Could you check a few things on this drawing? It's one solid part, dimensions in mm from its lowest x, y, z. A direction names the side the tool comes from. Round coordinates to 2 decimals unless told otherwise and drop trailing zeros. Write each loop counter-clockwise with the first axis right and the second up, starting at its lowest first coordinate (ties: lowest second). Pieces come first, ordered by that corner, then holes. Notation, with made-up numbers: M -3,-31 L 46,-31 A16 ccw 46,-16 Z; hole C 46,61 d10. An arc over 180 degrees is marked long. One line per item, written item: value. Start each with the question number.
(1) I want a section at C-C on y = 6. Please give me the cut outline in (x, z), and give its area (3 significant figures).
(2) Thinking about a two-plate mould opening in Z: for the marked faces 1, 2 and 3, which applies, released by +Z, released by -Z, zero draft, split by the parting line, or undercut?
(3) I want a section at B-B on z = 0.5. Please give me the cut outline in (x, y).
(4) I want a section at A-A on x = 9.75. Please give me the cut outline in (y, z).
(5) Which directions (+Z, -Z, +X, -X, +Y, -Y) give clear straight access to the entire face, cutting with the end or side of a thin tool? Please do the marked faces 4, 5 and 6.
(6) I want a section at D-D on z = 8.25. Please give me the cut outline in (x, y), and give its area (3 significant figures).
(7) I'm going to push flat-ended pins straight in: pin 1 Ø1.5 at (x, y) = (6, 5.5) entering from -Z; pin 2 Ø2 at (y, z) = (2, 7.5) entering from +X; pin 3 Ø2 at (x, z) = (1.5, 4.5) entering from +Y. Where does each tip first touch, or does it pass through?
(8) If I drill on L1, parallel to Y at x = 5.5, z = 4; L2, parallel to Y at x = 5.5, z = 1.5; L3, parallel to Z at x = 9, y = 6.5, over which ranges is the centre line in solid material (lowest first)?
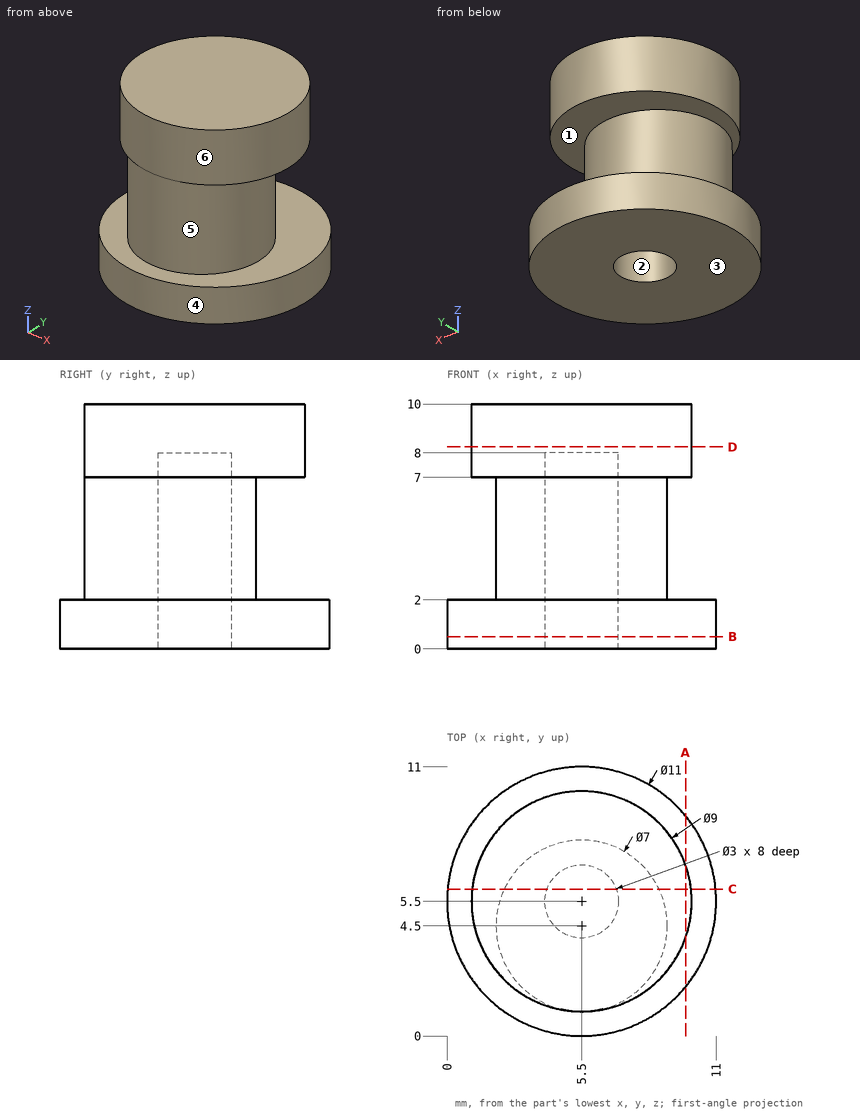
Found:
1. outline: M 0.02,0 L 4.09,0 L 4.09,8 L 6.91,8 L 6.91,0 L 10.98,0 L 10.98,2 L 8.66,2 L 8.66,7 L 9.97,7 L 9.97,10 L 1.03,10 L 1.03,7 L 2.34,7 L 2.34,2 L 0.02,2 Z
1. area: 57.7 mm²
2. face 1: undercut
2. face 2: zero draft
2. face 3: released by -Z
3. outline: C 5.5,5.5 d11; hole C 5.5,5.5 d3
4. outline: M 2.01,0 L 8.99,0 L 8.99,2 L 2.01,2 Z; M 4.02,7 L 6.98,7 L 6.98,10 L 4.02,10 Z
5. face 4: +Z, -Z
5. face 5: none
5. face 6: +Z
6. outline: C 5.5,5.5 d9
6. area: 63.6 mm²
7. pin 1: stops at z = 8
7. pin 2: stops at x = 9.24
7. pin 3: stops at y = 6.3
8. L1: y = 1 to 4, 7 to 8
8. L2: y = 0 to 4, 7 to 11
8. L3: z = 0 to 2, 7 to 10
